Verification items for this drawing (mm, ordinates from the low corner). Round coordinates to 2 decimals unless told otherwise and drop trailing zeros. Order: outer loops, then holes, each group sorted by start corner. A loop starts at its lowest first (then second) coordinate and runs counter-clockwise, first axis right, second up. Notation, with made-up numbers: (2.25, 76.5) - (60.25, 76.5) arc R15 ccw to (60.25, 96.5) - close; hole circle Ø3 at (20.5, 21). An arc over 180 degrees is marked (long way). One line per question, with ' | ' between items. Start each with the question number.
Q1. Gauge pin test, flat end, axial feed: P1, Ø1, axis at x = 2, y = 1, coming from the -Z side. Record the tip position at first contact, or that the pin passes through.
Q2. Sectioned sample at D-D, the plane x = 5.4. Enter the section's corners in (y, z), then the cut area to 3 significant figures.
Q3. Sectioned sample at A-A, the plane z = 53. Enter the section's corners in (x, y).
Q4. Material ranges on line 1 along Z through (x, y) = (3, 1.65); line 2 along Z through (x, y) = (3.6, 1.05); line 3 along X through (y, z) = (0.6, 13), recorded low to high.
Q5. Sectioned sample at B-B, the plane x = 3. Enter the section's corners in (y, z).
Q6. Sectioned sample at C-C, the plane y = 0.8. Enter the section's corners in (x, z).
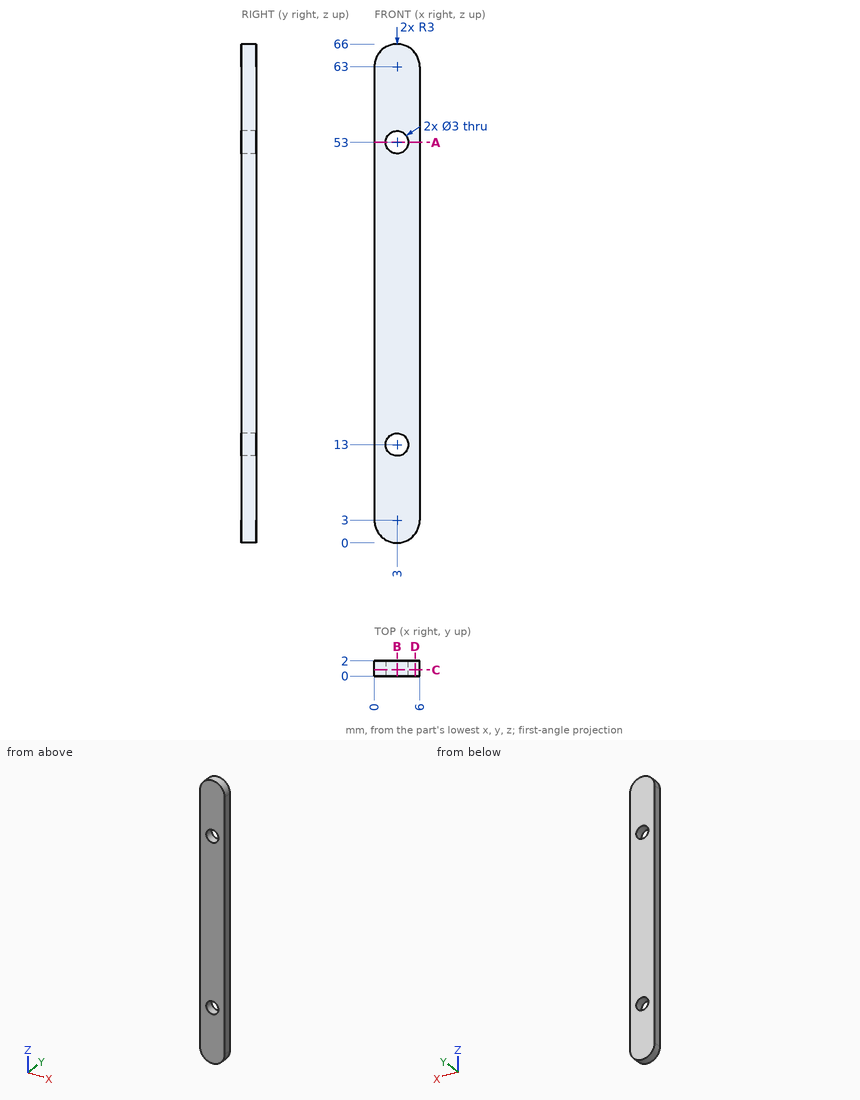
Determined:
1) P1: stops at z = 0.04
2) outline: (0, 1.2) - (2, 1.2) - (2, 64.8) - (0, 64.8) - close | area: 127 mm2
3) outline: (0, 0) - (1.5, 0) - (1.5, 2) - (0, 2) - close; (4.5, 0) - (6, 0) - (6, 2) - (4.5, 2) - close
4) line 1: z = 0 to 11.5, 14.5 to 51.5, 54.5 to 66 | line 2: z = 0.06 to 11.63, 14.37 to 51.63, 54.37 to 65.94 | line 3: x = 0 to 1.5, 4.5 to 6
5) outline: (0, 0) - (2, 0) - (2, 11.5) - (0, 11.5) - close; (0, 14.5) - (2, 14.5) - (2, 51.5) - (0, 51.5) - close; (0, 54.5) - (2, 54.5) - (2, 66) - (0, 66) - close
6) outline: (0, 3) arc R3 ccw to (6, 3) - (6, 63) arc R3 ccw to (0, 63) - close; hole circle Ø3 at (3, 13); hole circle Ø3 at (3, 53)
